from build123d import *

# Parameters (mm, degrees)
SKETCH004_R  = 2.5
PAD004_DEPTH = 5
SKETCH005_R  = 4.2
PAD005_DEPTH = 2
FILLET_R     = 0.5


with BuildPart() as part:
    # Sketch004 → Pad004 (new body)
    with BuildSketch(Plane.XY.offset(2)):
        with Locations((39.321, 17.435)):
            Circle(SKETCH004_R)
    extrude(amount=-PAD004_DEPTH)

    # Sketch005 → Pad005 (join)
    with BuildSketch(Plane.XY.offset(2)):
        with Locations((39.321, 17.435)):
            Circle(SKETCH005_R)
    extrude(amount=PAD005_DEPTH)

    # Fillet
    fillet_edges = [part.edges().sort_by_distance(p)[0] for p in [
        (36.821, 17.435, -3),
    ]]
    fillet(fillet_edges, radius=FILLET_R)


solid = part.part
The model under review builds one solid part; all positions refer to its coordinate system, in mm. A direction names the side the tool comes from. Coordinates: 2 decimals unless noted, no trailing zeros. Write each loop counter-clockwise with the first axis right and the second up, starting at its lowest first coordinate (ties: lowest second). Pieces come first, ordered by that corner, then holes. Notation, with made-up numbers: (76, 39.5) - (115, 39.5) arc R9 cw to (115, 55.5) - close; hole circle Ø10 at (-27.75, 76). An arc over 180 degrees is marked (long way). Answer as a JSON object with one key per item and string values. Group by question number.
1. To check wall thickness, follow probe 1 along Z at (x, y) = (42.25, 14.75); probe 2 along Y at (x, z) = (36, 3.25); probe 3 along X at (y, z) = (16.75, 0.5). State the ranges of each line that lie inside material, in increasing order.
2. Add section D-D (z = 2.5). Give the boundary of the cut face in (x, y) (3 decimals), plus the area to 3 significant figures.
3. Add section A-A (z = -0.75). Give the boundary of the cut face in (x, y) (3 decimals), plus the area to 3 significant figures.
4. Clearance check with flat-ended pins moving along their axes: pin 1 Ø1 at (x, z) = (42, 3) entering from +Y; pin 2 Ø1.5 at (x, z) = (38, 1) entering from -Y; pin 3 Ø3 at (x, z) = (41, -2) entering from -Y. State where each tip first meets the part, or that it passes through.
5. Add section B-B (x = 42.25). Give the boundary of the cut face in (y, z).
6. Machinability: for faces 1 (the face through (39.3, 14.7, 2)), 2 (the face through (39, 17, -3)), which of the approach directions +Z, -Z, +X, -X, +Y, -Y give a long, thin tool a straight path to every point of the face, cutting with its end or side? Answer none if there is none.
7. Add section C-C (y = 14). Give the boundary of the cut face in (x, z), plus the area to 3 significant figures.
Findings:
{
 "1": {"probe 1": "2 to 4", "probe 2": "14.86 to 20.01", "probe 3": "36.92 to 41.73"},
 "2": {"outline": "circle Ø8.4 at (39.321, 17.435)", "area": "55.4 mm²"},
 "3": {"outline": "circle Ø5 at (39.321, 17.435)", "area": "19.6 mm²"},
 "4": {"pin 1": "y = 21.03", "pin 2": "y = 15", "pin 3": "y = 14.94"},
 "5": {"outline": "(14.42, 2) - (20.45, 2) - (20.45, 4) - (14.42, 4) - close"},
 "6": {"face 1": "-Z", "face 2": "-Z, +X, -X, +Y, -Y"},
 "7": {"outline": "(36.9, 2) - (41.74, 2) - (41.74, 4) - (36.9, 4) - close", "area": "9.67 mm²"}
}
